Autodesk Inventor part; units mm, degrees
ref_plane "Plan YZ" through (0, 0, 0) normal (1, 0, 0) x (0, 1, 0)
ref_plane "Plan XZ" through (0, 0, 0) normal (0, 1, 0) x (-1, 0, 0)
ref_plane "Plan XY" through (0, 0, 0) normal (0, 0, 1) x (1, 0, 0)
sketch "Esquisse7" plane through (0, 0, 0) normal (0, 0, 1) x (1, 0, 0)
  line L0 (-86, -26) -> (-86, 26)
  line L1 (-86, 26) -> (-81, 26)
  line L2 (-81, 26) -> (-81, 29)
  line L3 (-81, 29) -> (-66, 29)
  line L4 (-66, 29) -> (-66, 26)
  line L5 (-66, 26) -> (-7.5, 26)
  line L6 (-7.5, 26) -> (-7.5, 29)
  line L7 (-7.5, 29) -> (7.5, 29)
  line L8 (7.5, 29) -> (7.5, 26)
  line L9 (7.5, 26) -> (66, 26)
  line L10 (66, 26) -> (66, 29)
  line L11 (66, 29) -> (81, 29)
  line L12 (81, 29) -> (81, 26)
  line L13 (81, 26) -> (86, 26)
  line L14 (86, 26) -> (86, -26)
  line L15 (86, -26) -> (81, -26)
  line L16 (81, -26) -> (81, -29)
  line L17 (81, -29) -> (66, -29)
  line L18 (66, -29) -> (66, -26)
  line L19 (7.5, -26) -> (7.5, -29)
  line L20 (7.5, -26) -> (66, -26)
  line L21 (7.5, -29) -> (-7.5, -29)
  line L22 (-7.5, -29) -> (-7.5, -26)
  line L23 (-7.5, -26) -> (-66, -26)
  line L24 (-66, -26) -> (-66, -29)
  line L25 (-66, -29) -> (-81, -29)
  line L26 (-81, -29) -> (-81, -26)
  line L27 (-81, -26) -> (-86, -26)
  line L28 (0, -40.6) -> (0, 40.6) construction
  line L29 (-120.4, 0) -> (120.4, 0) construction
  dimension "d33" = 52
  dimension "d34" = 15
  dimension "d35" = 3
  dimension "d36" = 5
  dimension "d65" = 172
extrude "Extrusion2" add sketch "Esquisse7" against normal blind 3
sketch "Esquisse8" plane through (0, 0, 0) normal (0, 0, 1) x (1, 0, 0)
  point P0 (0, 0)
  point P1 (7.5, 26)
  point P2 (-7.5, 26)
  point P3 (-81, 26)
  point P4 (-66, 26)
  point P5 (-81, -26)
  point P6 (-66, -26)
  point P7 (-7.5, -26)
  point P8 (7.5, -26)
  point P9 (66, -26)
  point P10 (81, -26)
  point P11 (66, 26)
  point P12 (81, 26)
  point P13 (81, 26)
  point P14 (66, -26)
  point P15 (81, 26)
hole "Perçage2" at (7.5, 26, 0) at (-7.5, 26, 0) at (-81, 26, 0) at (-66, 26, 0) at (-81, -26, 0) at (-66, -26, 0) at (-7.5, -26, 0) at (7.5, -26, 0) at (66, -26, 0) at (81, -26, 0) at (66, 26, 0) at (81, 26, 0) direction (0, 0, -1) diameter 1 end through all
sketch "Esquisse9" plane through (0, 0, 0) normal (0, 0, 1) x (1, 0, 0)
  circle A0 centre (-24, 13.8) radius 4.5
  line L0 (-86, -26) -> (-86, 26)
  line L1 (-65.5, 26) -> (-8, 26)
  point P0 (0, 0)
  point P1 (-90, -24)
  point P2 (-90, 24)
  dimension "d62" = 62
  dimension "d63" = 12.2
  dimension "d64" = 9
extrude "Extrusion3" cut sketch "Esquisse9" against normal through all
chamfer "Chanfrein3" distance 1 angle 45 12 edges at (-81, -29, -1.5) (-66, -29, -1.5) (-81, 29, -1.5) (-66, 29, -1.5) (-7.5, 29, -1.5) (7.5, 29, -1.5) (66, 29, -1.5) (81, 29, -1.5) (66, -29, -1.5) (81, -29, -1.5) (-7.5, -29, -1.5) (7.5, -29, -1.5)
properties part number "P1704_202" material "Plastique PMMA"
Part model, mm, in its own coordinate system. A direction names the side the tool comes from. Give positions to 0.01 mm unless a question says otherwise; leave off trailing zeros. Order: outer loops, then holes, each group sorted by start corner. A loop starts at its lowest first (then second) coordinate and runs counter-clockwise, first axis right, second up. Notation, with made-up numbers: M 6,74.5 L 33,74.5 A18 cw 33,101.5 Z; hole C 80,16 d1. An arc over 180 degrees is marked long. Use a Markdown table: item, result. Add a question column.
(1) 3-axis set-ups, long thin cutter, end or side, ignore diameter. For faces 5 (the face through (-84, -26, -1)), 6 (the face through (-36, -26, -1)), 7 (the face through (84, 26, -1)): which of +Z, -Z, +X, -X, +Y, -Y reach the whole face in a straight line?
(2) Drop flat-ended pins along their axis: P1, Ø1.2, axis at y = -27, z = -1, coming from the -X side; P2, Ø1.6, axis at y = 27.5, z = -2, coming from the +X side; P3, Ø0.9, axis at x = 83, z = -2, coming from the -Y side; P4, Ø10, axis at x = -68.5, y = 19.5, coming from the +Z side. Give the stop position or say it passes through.
(3) Probe line 1 along Y through (x, z) = (-51, -0.55). List the from-to ranges inside material, lowest first. Write a range as [from, to].
(4) Mould opens along X. For faces 1 (the face through (-84, 26, -1)), 2 (the face through (36, 26, -1)), 3 (the face through (86, 0, -1)), 4 (the face through (-86, 0, -1)) say: +X half, -X half, draft (parallel to the pull), parting line (faces both ways), or undercut.
(5) Saw through at A-A, the plane y = 13.8. Give the cut face in (x, z).
Answer key:
| question | item | result |
|---|---|---|
| 1 | face 5 | +Z, -Z, -X, -Y |
| 1 | face 6 | +Z, -Z, -Y |
| 1 | face 7 | +Z, -Z, +X, +Y |
| 2 | P1 | x = -81 |
| 2 | P2 | x = 81 |
| 2 | P3 | y = -26 |
| 2 | P4 | z = 0 |
| 3 | line 1 | [-26, 26] |
| 4 | face 1 | draft |
| 4 | face 2 | undercut |
| 4 | face 3 | +X half |
| 4 | face 4 | -X half |
| 5 | outline | M -86,-3 L -28.5,-3 L -28.5,0 L -86,0 Z; M -19.5,-3 L 86,-3 L 86,0 L -19.5,0 Z |
